```python
from build123d import *

# Parameters (mm, degrees)
BOSS_EXTRUDE1_DEPTH = 5.715
SKETCH3_R           = 1.25
SKETCH3_R_2         = 1
SKETCH3_R_3         = 1.5
CUT_EXTRUDE1_DEPTH  = 5.715


with BuildPart() as part:
    # Sketch1 → Boss-Extrude1 (new body)
    with BuildSketch(Plane.XY):
        Polygon((-37.8206, -20.2565), (-37.8206, 20.2565), (-31.75, 20.2565), (-31.75, 39.0525), (-25.4, 60.6425), (25.4, 60.6425), (31.75, 39.0525), (31.75, 20.2565), (37.8206, 20.2565), (37.8206, -20.2565), (29.21, -34.6075), (29.21, -57.4675), (-29.21, -57.4675), (-29.21, -34.6075), align=None)
    extrude(amount=BOSS_EXTRUDE1_DEPTH)

    # Sketch3 → Cut-Extrude1 (cut)
    with BuildSketch(Plane.XY.offset(5.715)):
        with Locations((-24.5, 10.6925)):
            Circle(SKETCH3_R)
        with Locations((24.5, 10.6925)):
            Circle(SKETCH3_R)
        with Locations((-24.5, -47.3075)):
            Circle(SKETCH3_R)
        with Locations((24.5, -47.3075)):
            Circle(SKETCH3_R)
        with Locations((0, 55.5625)):
            Circle(SKETCH3_R_2)
        with Locations((17.5, 30.5625)):
            Circle(SKETCH3_R_2)
        with Locations((-17.5, 30.5625)):
            Circle(SKETCH3_R_2)
        with Locations((-17.5, -54.4375)):
            Circle(SKETCH3_R_2)
        with Locations((17.5, -54.4375)):
            Circle(SKETCH3_R_2)
        with Locations((-15.7, 57.48249997)):
            Circle(SKETCH3_R_3)
        with Locations((15.7, 57.48249997)):
            Circle(SKETCH3_R_3)
        with Locations((15.7, 43.48249997)):
            Circle(SKETCH3_R_3)
        with Locations((-15.7, 43.48249997)):
            Circle(SKETCH3_R_3)
    extrude(amount=-CUT_EXTRUDE1_DEPTH, mode=Mode.SUBTRACT)


solid = part.part
```
Design review of the part built by this model. Coordinates are the model's own, in mm. A direction names the side the tool comes from. Coordinates: 2 decimals unless noted, no trailing zeros. Write each loop counter-clockwise with the first axis right and the second up, starting at its lowest first coordinate (ties: lowest second). Pieces come first, ordered by that corner, then holes.
1) Machinability: for faces 1 (the flat face through (-31.75, 30, 3)), 2 (the cylindrical face through (-14.894, 58.747, 2.898)), 3 (the flat face through (-29.21, -46, 3)), which of the approach directions +Z, -Z, +X, -X, +Y, -Y give a long, thin tool a straight path to every point of the face, cutting with its end or side? Answer none if there is none.
2) Mouldability with a two-part tool opening along X and no side actions: class faces 4 (the flat face through (28.53, 50, 2.82)), 5 (the flat face through (35, 20.256, 3)), 6 (the cylindrical face through (-24.663, -46.068, 2.898)) as +X half, -X half, draft (parallel to the pull), parting line (faces both ways), or undercut.
3) Add section B-B (y = 47). Write out the cut boundary in (x, z) (1 decimal).
4) Add section A-A (z = 1.3). State how many separate pieces and enclosed holes the cut face has, plus the area to 3 significant figures.
5) Insertion check: pin 1 (1.7 mm diameter, centred on x = 36.5, z = 3, fed in from +Y); pin 2 (3 mm diameter, centred on y = -41, z = 1.5, fed in from +X); pin 3 (3 mm diameter, centred on y = 29.5, z = 4, fed in from +X). Each pin has a flat end and moves straight along its axis. Give the tip position at first contact, or say it passes through.
6) To check wall thickness, follow L1, parallel to Y at x = -24.5, z = 1.8; L2, parallel to Y at x = 17.5, z = 3.3; L3, parallel to X at y = 11.5, z = 3.5. State the ranges of each line that lie inside material, in increasing order.
Check result:
1. face 1: +Z, -Z, -X, +Y
1. face 2: +Z, -Z
1. face 3: +Z, -Z, -X, -Y
2. face 4: +X half
2. face 5: draft
2. face 6: undercut
3. outline: (-29.4, 0) - (29.4, 0) - (29.4, 5.7) - (-29.4, 5.7) - close
4. separate pieces: 1
4. enclosed holes: 13
4. area: 7,730 mm2
5. pin 1: stops at y = 20.26
5. pin 2: stops at x = 29.21
5. pin 3: stops at x = 31.75
6. L1: y = -57.47 to -48.56, -46.06 to 9.44, 11.94 to 60.64
6. L2: y = -57.47 to -55.44, -53.44 to 29.56, 31.56 to 60.64
6. L3: x = -37.82 to -25.45, -23.55 to 23.55, 25.45 to 37.82
